```python
from build123d import *

# Parameters (mm, degrees)
SM_BASE_FLANGE_1_DEPTH   = 15
OTHER_START              = -24.748737342
OTHER_1_OUTLINE_W        = 1.5
OTHER_1_OUTLINE_H        = 23.213203436
OTHER_1_DEPTH            = 3.535533906
OTHER_START_2            = -7.071067812
OTHER_1_2_OUTLINE_W      = 1.5
OTHER_1_2_OUTLINE_H      = 3.786796564
OTHER_1_2_DEPTH          = 7.071067812
SKETCH_6_R               = 5.5
CUT_EXTRUDE_734_DEPTH    = 78.162166896
SKETCH_8_W               = 67
SKETCH_8_H               = 26
SM_BASE_FLANGE_1_2_DEPTH = 1.5
SKETCH_7_R               = 2.5
CUT_EXTRUDE_2_DEPTH      = 10


# Read off the part's stored shape, not the designer's step: Затупленный угол1
# Sheet-metal steps are written as plain solids
with BuildPart() as part:
    # Sketch 1 → Sm Base Flange 1 (new, symmetric)
    with BuildSketch(Plane.XY):
        with BuildLine():
            Line((-35, -20), (-35, -1.5))
            ThreePointArc((-35, -1.5), (-34.560660172, -0.439339828), (-33.5, 0))
            Line((-33.5, 0), (33.5, 0))
            ThreePointArc((33.5, 0), (34.560660172, -0.439339828), (35, -1.5))
            Line((35, -1.5), (35, -20))
            Line((35, -20), (36.5, -20))
            Line((36.5, -20), (36.5, -1.5))
            ThreePointArc((36.5, -1.5), (35.621320344, 0.621320344), (33.5, 1.5))
            Line((33.5, 1.5), (-33.5, 1.5))
            ThreePointArc((-33.5, 1.5), (-35.621320344, 0.621320344), (-36.5, -1.5))
            Line((-36.5, -1.5), (-36.5, -20))
            Line((-36.5, -20), (-35, -20))
        make_face()
    extrude(amount=SM_BASE_FLANGE_1_DEPTH, both=True)

    # Other 1 outline → Other 1 (cut)
    with BuildSketch(Plane(origin=(0, 0, 0), x_dir=(1, 0, 0), z_dir=(0, 0.707106781186548, -0.707106781186547)).offset(OTHER_START)):
        with Locations((-35.75, 9.606601718)):
            Rectangle(OTHER_1_OUTLINE_W, OTHER_1_OUTLINE_H)
        with Locations((35.75, 9.606601718)):
            Rectangle(OTHER_1_OUTLINE_W, OTHER_1_OUTLINE_H)
    extrude(amount=OTHER_1_DEPTH, mode=Mode.SUBTRACT)

    # Other 1 2 outline → Other 1 2 (cut)
    with BuildSketch(Plane(origin=(0, 0, 0), x_dir=(1, 0, 0), z_dir=(0, 0.707106781186548, -0.707106781186547)).offset(OTHER_START_2)):
        with Locations((-35.75, 23.106601718)):
            Rectangle(OTHER_1_2_OUTLINE_W, OTHER_1_2_OUTLINE_H)
        with Locations((35.75, 23.106601718)):
            Rectangle(OTHER_1_2_OUTLINE_W, OTHER_1_2_OUTLINE_H)
    extrude(amount=OTHER_1_2_DEPTH, mode=Mode.SUBTRACT)

    # Эскиз6 → Cut-Extrude 734 (cut, through all)
    with BuildSketch(Plane.ZY.offset(36.5)):
        with Locations((0, -10)):
            Circle(SKETCH_6_R)
    extrude(amount=-CUT_EXTRUDE_734_DEPTH, mode=Mode.SUBTRACT)

    # Эскиз8 → Sm Base Flange 1 2 (add)
    with BuildSketch(Plane(origin=(0, 1.5, 0), x_dir=(1, 0, 0), z_dir=(0, 1, 0))):
        with Locations((0, -28)):
            Rectangle(SKETCH_8_W, SKETCH_8_H)
    extrude(amount=-SM_BASE_FLANGE_1_2_DEPTH)

    # Эскиз7 → Вырез-Вытянуть2 (cut)
    with BuildSketch(Plane(origin=(0, 1.5, 0), x_dir=(1, 0, 0), z_dir=(0, 1, 0))):
        with Locations(Location((-20, -26, 0), (0, 0, 270))):
            Circle(SKETCH_7_R)
        with Locations(Location((20, -26, 0), (0, 0, 90))):
            Circle(SKETCH_7_R)
    extrude(amount=-CUT_EXTRUDE_2_DEPTH, mode=Mode.SUBTRACT)


solid = part.part
```
The model under review builds one solid part; all positions refer to its coordinate system, in mm. A direction names the side the tool comes from. Round coordinates to 2 decimals unless told otherwise and drop trailing zeros. Loops run counter-clockwise (first coordinate to the right, second up) from the corner with the lowest first, then second, coordinate; pieces in that order, holes last. Notation, with made-up numbers: M 54.5,68.5 L 80.5,68.5 A22 ccw 80.5,76.5 Z; hole C -16,18 d11. An arc over 180 degrees is marked long. Answer as a JSON object with one key per item and string values.
(1) Draft analysis for pull direction X (two halves, no side actions). For faces 1 (the flat face through (-33.5, 1, 28)), 2 (the flat face through (36.5, -15, 4)), 3 (the cylindrical face through (18.31, 0.76, 27.84)), 4 (the flat face through (36, -18, -12)), state which applies: released by +X, released by -X, zero draft, split by the parting line, or undercut.
Resolved:
{"face 1": "released by -X", "face 2": "released by +X", "face 3": "undercut", "face 4": "zero draft"}
(2) Take a section at B-B on x = 20. Give the boundary of the cut face in (y, z), and give its area (3 significant figures).
Resolved:
{"outline": "M 0,-15 L 1.5,-15 L 1.5,23.5 L 0,23.5 Z; M 0,28.5 L 1.5,28.5 L 1.5,41 L 0,41 Z", "area": "76.5 mm²"}
(3) Take a section at D-D on z = 0. Give the boundary of the cut face in (x, y), and give its area (3 significant figures).
Resolved:
{"outline": "M -36.5,-20 L -35,-20 L -35,-15.5 L -36.5,-15.5 Z; M -36.5,-4.5 L -35,-4.5 L -35,-1.5 A1.5 cw -33.5,0 L 33.5,0 A1.5 cw 35,-1.5 L 35,-4.5 L 36.5,-4.5 L 36.5,-1.5 A3 ccw 33.5,1.5 L -33.5,1.5 A3 ccw -36.5,-1.5 Z; M 35,-20 L 36.5,-20 L 36.5,-15.5 L 35,-15.5 Z", "area": "134 mm²"}
(4) Take a section at C-C on y = -10. Give the boundary of the cut face in (x, z).
Resolved:
{"outline": "M -36.5,-15 L -35,-15 L -35,-5.5 L -36.5,-5.5 Z; M -36.5,5.5 L -35,5.5 L -35,15 L -36.5,15 Z; M 35,-15 L 36.5,-15 L 36.5,-5.5 L 35,-5.5 Z; M 35,5.5 L 36.5,5.5 L 36.5,15 L 35,15 Z"}
(5) Take a section at A-A on z = 27.5. Give the boundary of the cut face in (x, y), and give its area (3 significant figures).
Resolved:
{"outline": "M -33.5,0 L -22,0 L -22,1.5 L -33.5,1.5 Z; M -18,0 L 18,0 L 18,1.5 L -18,1.5 Z; M 22,0 L 33.5,0 L 33.5,1.5 L 22,1.5 Z", "area": "88.5 mm²"}
(6) Tool access review of faces 5 (the flat face through (36, -18, 12)), 6 (the flat face through (33.5, 1, 28)), 7 (the flat face through (0, 0, 13)): name each direction out of +Z, -Z, +X, -X, +Y, -Y from which nothing blocks a thin tool from reaching the whole face with its end or side.
Resolved:
{"face 5": "+Z, +X, -X, -Y", "face 6": "+Z, +X, +Y, -Y", "face 7": "+Z, -Z, -Y"}
(7) To check wall thickness, follow line 1 along X through (y, z) = (1, 26); line 2 along X through (y, z) = (-3.5, -1); line 3 along Z through (x, y) = (20, 0.55). State the ranges of each line that lie inside material, in increasing order.
Resolved:
{"line 1": "-33.5 to -22.5, -17.5 to 17.5, 22.5 to 33.5", "line 2": "-36.5 to -35, 35 to 36.5", "line 3": "-15 to 23.5, 28.5 to 41"}
(8) Clearance check with flat-ended pins moving along their axes: P1, Ø3.5, axis at x = -35, y = -7.5, coming from the +Z side; P2, Ø8, axis at x = 17.5, y = -3.5, coming from the -Z side; P3, Ø2, axis at x = -8.5, z = 30, coming from the -Y side; P4, Ø1.6, axis at y = 0.5, z = 31.5, coming from the +X side. State where each tip first meets the part, or that it passes through.
Resolved:
{"P1": "z = 15", "P2": "z = -15", "P3": "y = 0", "P4": "x = 33.5"}
